Could you check a few things on this model? Use its own coordinates, in mm. Give positions to 0.01 mm unless a question says otherwise; leave off trailing zeros. Loops run counter-clockwise (first coordinate to the right, second up) from the corner with the lowest first, then second, coordinate; pieces in that order, holes last. Notation, with made-up numbers: (77, -22.75) - (109, -22.75) arc R25 cw to (109, -0.75) - close; hole circle Ø4 at (-10, 74.25). An arc over 180 degrees is marked (long way). Write each question's results on one line, items separated by ' | '. Start each with the question number.
1) I want a section at A-A, the plane x = -22.5. Write out the boundary of the cut face in (y, z).
2) I want a section at D-D, the plane x = 21. Write out the boundary of the cut face in (y, z).
3) I'm going to push a flat-ended pin straight in: pin 1 (1.5 mm diameter, centred on x = -20, z = -1, fed in from +Y). Where does the tip first touch, or does it pass through?
4) If we mould it in two halves opening along X, with no side actions, what happens to faces 1 (the face through (-36, -5, 0)), 2 (the face through (-1, -5, -4.5)), 3 (the face through (10.083, -4.93, -0.759))? For each: +X half, -X half, draft (parallel to the pull), parting line (faces both ways), or undercut.
5) If I drill on probe 1 along Z at (x, y) = (7, -8); probe 2 along Z at (x, y) = (21, -5.5), over which ranges is the centre line in solid material (lowest first)? Write a range as [from, to].
6) I want a section at B-B, the plane y = -9.25. Count the separate pieces of the cut face and the enclosed holes in it, and give its area (3 significant figures).
from build123d import *

# Parameters (mm, degrees)
SKETCH1_W           = 72
SKETCH1_H           = 9
SKETCH1_R           = 3.5
BOSS_EXTRUDE1_DEPTH = 10


with BuildPart() as part:
    # Sketch1 → Boss-Extrude1 (new body)
    with BuildSketch(Plane(origin=(0, 0, 0), x_dir=(1, 0, 0), z_dir=(0, 1, 0))):
        Rectangle(SKETCH1_W, SKETCH1_H)
        with Locations(Location((-4.5, 0, 0), (0, 0, 270))):
            Circle(SKETCH1_R, mode=Mode.SUBTRACT)
        with Locations(Location((4.5, 0, 0), (0, 0, 270))):
            Circle(SKETCH1_R, mode=Mode.SUBTRACT)
        with Locations(Location((13.5, 0, 0), (0, 0, 270))):
            Circle(SKETCH1_R, mode=Mode.SUBTRACT)
        with Locations(Location((22.5, 0, 0), (0, 0, 270))):
            Circle(SKETCH1_R, mode=Mode.SUBTRACT)
        with Locations(Location((31.5, 0, 0), (0, 0, 270))):
            Circle(SKETCH1_R, mode=Mode.SUBTRACT)
        with Locations(Location((-13.5, 0, 0), (0, 0, 270))):
            Circle(SKETCH1_R, mode=Mode.SUBTRACT)
        with Locations(Location((-22.5, 0, 0), (0, 0, 270))):
            Circle(SKETCH1_R, mode=Mode.SUBTRACT)
        with Locations(Location((-31.5, 0, 0), (0, 0, 270))):
            Circle(SKETCH1_R, mode=Mode.SUBTRACT)
    extrude(amount=-BOSS_EXTRUDE1_DEPTH)


solid = part.part
Answers:
1) outline: (-10, -4.5) - (0, -4.5) - (0, -3.5) - (-10, -3.5) - close; (-10, 3.5) - (0, 3.5) - (0, 4.5) - (-10, 4.5) - close
2) outline: (-10, -4.5) - (0, -4.5) - (0, -3.16) - (-10, -3.16) - close; (-10, 3.16) - (0, 3.16) - (0, 4.5) - (-10, 4.5) - close
3) pin 1: passes through
4) face 1: -X half | face 2: draft | face 3: undercut
5) probe 1: z = [-4.5, -2.45], [2.45, 4.5] | probe 2: z = [-4.5, -3.16], [3.16, 4.5]
6) separate pieces: 1 | enclosed holes: 8 | area: 340 mm2
